Verification items for this drawing (mm, ordinates from the low corner). A direction names the side the tool comes from. Round coordinates to 2 decimals unless told otherwise and drop trailing zeros. Order: outer loops, then holes, each group sorted by start corner. A loop starts at its lowest first (then second) coordinate and runs counter-clockwise, first axis right, second up. Notation, with made-up numbers: (71.25, 88) -> (91.25, 88) arc R30 cw to (91.25, 113) -> close; hole circle Ø5 at (-9.75, 85.5). An arc over 180 degrees is marked (long way). Answer in a Markdown table with one row per item.
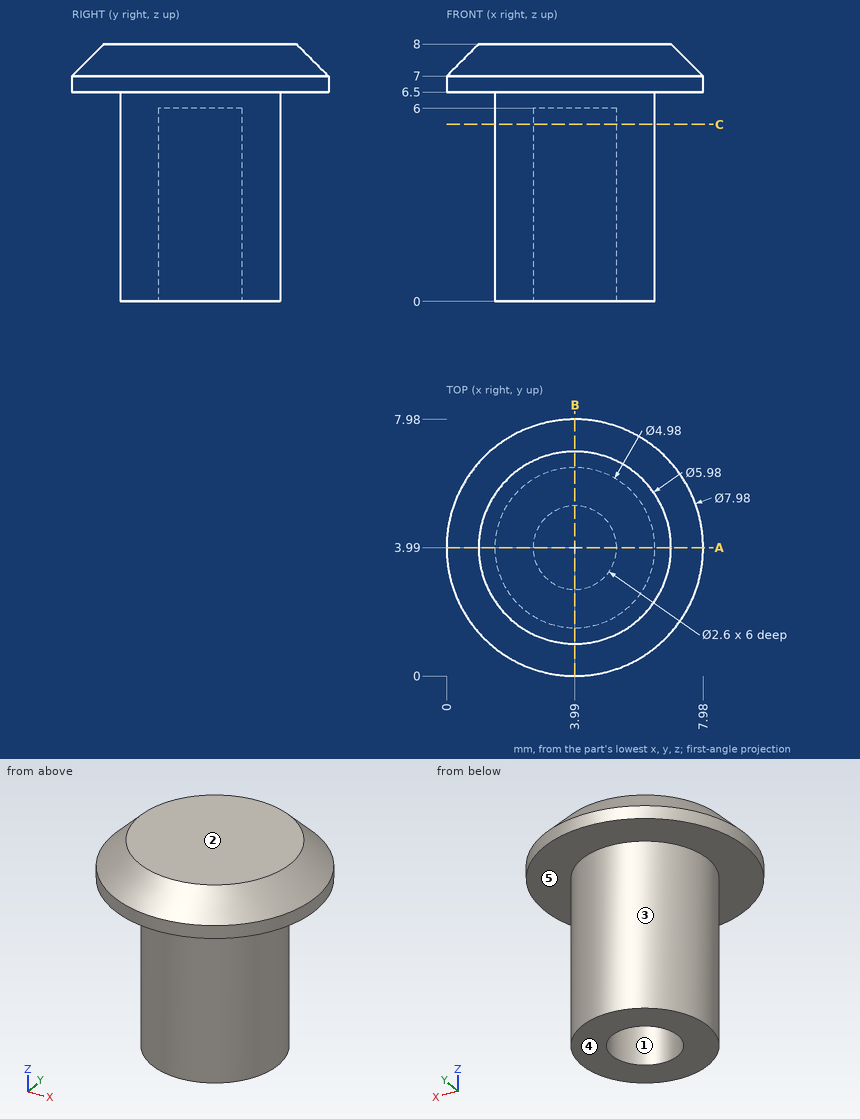
Item 1: Scan lines: line 1 (X direction, y = 4, z = 2); line 2 (Z direction, x = 1.5, y = 3.25). Record each from-to range of solid material in increasing order. Write a range as [from, to].
Result sheet:
| item | result |
|---|---|
| line 1 | x = [1.5, 2.69], [5.29, 6.48] |
| line 2 | z = [6.5, 8] |
Item 2: Cross-section at C-C (z = 5.5). Record the boundary of the cut face in (x, y), and give its area (3 significant figures).
Result sheet:
| item | result |
|---|---|
| outline | circle Ø4.98 at (3.99, 3.99); hole circle Ø2.6 at (3.99, 3.99) |
| area | 14.2 mm^2 |
Item 3: Mould release check, pull along Y, two halves, no side actions. Record for the marked faces 1, 2 and 3: pulls with the +Y half, pulls with the -Y half, needs draft (parallel to the pull), parting line crosses it, or undercut.
Result sheet:
| item | result |
|---|---|
| face 1 | undercut |
| face 2 | needs draft |
| face 3 | parting line crosses it |
Item 4: Cross-section at A-A (y = 3.99). Record the boundary of the cut face in (x, z).
Result sheet:
| item | result |
|---|---|
| outline | (0, 6.5) -> (1.5, 6.5) -> (1.5, 0) -> (2.69, 0) -> (2.69, 6) -> (5.29, 6) -> (5.29, 0) -> (6.48, 0) -> (6.48, 6.5) -> (7.98, 6.5) -> (7.98, 7) -> (6.98, 8) -> (1, 8) -> (0, 7) -> close |
Item 5: Set-up check for the marked faces 4 and 5: record each of +Z, -Z, +X, -X, +Y, -Y from which the full face is reachable in a straight line by a thin tool's end or side.
Result sheet:
| item | result |
|---|---|
| face 4 | -Z, +X, -X, +Y, -Y |
| face 5 | -Z |
Item 6: Depth check by flat-ended pin: P1, Ø2.5, axis at x = 3.99, y = 3.99, coming from the -Z side; P2, Ø4, axis at x = 6, y = 3, coming from the -Z side; P3, Ø1.5, axis at x = 7, y = 5.5, coming from the -Z side; P4, Ø1, axis at x = 2.5, z = 5.5, coming from the +Y side. Enter the tip coordinate at first touch or a pass-through.
Result sheet:
| item | result |
|---|---|
| P1 | stops at z = 6 |
| P2 | stops at z = 0 |
| P3 | stops at z = 6.5 |
| P4 | stops at y = 6.27 |
